Check sheet for the modelled part. Datum: model origin and axes. Units: mm. A direction names the side the tool comes from. Coordinates: 2 decimals unless noted, no trailing zeros. Loops run counter-clockwise (first coordinate to the right, second up) from the corner with the lowest first, then second, coordinate; pieces in that order, holes last. Notation, with made-up numbers: M 26.25,79.25 L 33.25,79.25 A29 ccw 33.25,116.25 Z; hole C -29.75,23 d11. An arc over 180 degrees is marked long. Answer in a Markdown table with one row per item. Add a question column.
Autodesk Inventor part; units mm, degrees
ref_plane "YZ Plane" through (0, 0, 0) normal (1, 0, 0) x (0, 1, 0)
ref_plane "XZ Plane" through (0, 0, 0) normal (0, 1, 0) x (-1, 0, 0)
ref_plane "XY Plane" through (0, 0, 0) normal (0, 0, 1) x (1, 0, 0)
sketch "Boceto1" plane through (0, 0, 0) normal (0, 0, 1) x (1, 0, 0)
  line L0 (-46, -14.91) -> (-46, -35.91)
  line L1 (-44.1, -31.91) -> (-2.9, -31.91)
  line L2 (-1, -35.91) -> (-1, -20.31)
  line L3 (-8.1, 6.6131) -> (-8.1, -14.91)
  line L4 (-44.6, -16.31) -> (-6.4, -16.31)
  line L5 (-2.4, -20.31) -> (-2.4, -30.01)
  line L6 (-2.9, -30.51) -> (-44.1, -30.51)
  line L7 (-44.6, -30.01) -> (-44.6, -16.31)
  arc A0 (-2.4, -20.31) -> (-6.4, -16.31) centre (-6.4, -20.31) ccw
  line L8 (-2.4, -32.41) -> (-2.4, -34.1632)
  line L9 (-3.5, -35.91) -> (-1, -35.91)
  line L10 (-9.5, -14.91) -> (-9.5, 7.7994)
  line L11 (-44.6, -32.41) -> (-44.6, -34.2323)
  line L12 (-43.5, -35.91) -> (-46, -35.91)
  line L13 (-43.5, -35.91) -> (-43.5, -35.4546)
  line L14 (-3.5, -35.91) -> (-3.5, -35.21)
  line L15 (-43.7447, -35.0247) -> (-44.3553, -34.6622)
  line L16 (-3.5, -35.21) -> (-2.6082, -34.5692)
  arc A1 (-2.9, -30.51) -> (-2.4, -30.01) centre (-2.9, -30.01) ccw
  arc A2 (-2.4, -32.41) -> (-2.9, -31.91) centre (-2.9, -32.41) ccw
  arc A3 (-2.6082, -34.5692) -> (-2.4, -34.1632) centre (-2.9, -34.1632) ccw
  arc A4 (-44.6, -30.01) -> (-44.1, -30.51) centre (-44.1, -30.01) ccw
  arc A5 (-44.1, -31.91) -> (-44.6, -32.41) centre (-44.1, -32.41) ccw
  arc A6 (-44.6, -34.2323) -> (-44.3553, -34.6622) centre (-44.1, -34.2323) ccw
  arc A7 (-43.5, -35.4546) -> (-43.7447, -35.0247) centre (-44, -35.4546) ccw
  line L17 (-9.5, 7.7994) -> (-4.75, 8.59)
  line L18 (-4.75, 8.59) -> (0, 7.7994)
  line L19 (-8.1, 6.6131) -> (-4.75, 7.1707)
  line L20 (-4.75, 7.1707) -> (-1.4, 6.6131)
  line L21 (0, 7.7994) -> (0, 0)
  line L22 (0, 0) -> (-1.4, 0)
  line L23 (-1.4, 0) -> (-1.4, 6.6131)
  line L24 (-8.1, -14.91) -> (-6.4, -14.91)
  arc A8 (-1, -20.31) -> (-6.4, -14.91) centre (-6.4, -20.31) ccw
  line L25 (-4.75, 16.5254) -> (-4.75, 0) construction
  line L26 (-38.9, 6.6131) -> (-38.9, -14.91)
  line L27 (-37.5, -14.91) -> (-37.5, 7.7994)
  line L28 (-37.5, 7.7994) -> (-42.25, 8.59)
  line L29 (-42.25, 8.59) -> (-47, 7.7994)
  line L30 (-38.9, 6.6131) -> (-42.25, 7.1707)
  line L31 (-42.25, 7.1707) -> (-45.6, 6.6131)
  line L32 (-47, 7.7994) -> (-47, 0)
  line L33 (-47, 0) -> (-45.6, 0)
  line L34 (-45.6, 0) -> (-45.6, 6.6131)
  line L35 (-42.25, 16.5254) -> (-42.25, 0) construction
  line L36 (-9.5, -14.91) -> (-37.5, -14.91)
  line L37 (-38.9, -14.91) -> (-46, -14.91)
  line L38 (-23.5, 14.1873) -> (-23.5, -36.7854) construction
  point P0 (-44.6, -34.5169)
  point P1 (-43.5, -35.17)
  dimension "d17" = 4
  dimension "d24" = 1.4
  dimension "d50" = 0.7
  dimension "d61" = 0.74
  dimension "d62" = 30.7
  dimension "d63" = 35.7
  dimension "d206" = 1.4
  dimension "d207" = 1.4
  dimension "d210" = 1.4
  dimension "d211" = 1.4
  dimension "d213" = 14.2
  dimension "d214" = 1.4
  dimension "d215" = 1.4
  dimension "d216" = 1.4
  dimension "d217" = 1.4
  dimension "d218" = 45
  dimension "d223" = 5.4
  dimension "d224" = 1.4
  dimension "d225" = 9.5
  dimension "d226" = 4.75
  dimension "d227" = 3.35
  dimension "d228" = 6.7
  dimension "d229" = 44.5
  dimension "d230" = 3.35
  dimension "d231" = 2.5
  dimension "d232" = 2.5
  dimension "d240" = 8.59
  dimension "d241" = 3.35
  dimension "d242" = 99.45
  dimension "d243" = 161.1
  dimension "d246" = 1.4
  dimension "d247" = 1.4
  dimension "d248" = 1.4
  dimension "d253" = 1.4
  dimension "d254" = 1.4
  dimension "d255" = 1.4
  dimension "d256" = 1.4
  dimension "d257" = 8.59
  dimension "d258" = 161.1
  dimension "d259" = 99.45
  dimension "d260" = 22.5
  dimension "d266" = 23.5
  dimension "d267" = 47
  dimension "d268" = 3.35
  dimension "d269" = 9.5
  dimension "d270" = 4.75
  dimension "d271" = 3.35
  dimension "d272" = 6.7
  dimension "d273" = 28
  dimension "d274" = 37.5
  dimension "d275" = 8.5
  dimension "d276" = 8.5
  dimension "d277" = 44.5
  dimension "d278" = 0.5
  dimension "d279" = 14.91
  dimension "d280" = 14.91
  dimension "d283" = 16.5254
  dimension "d284" = 0
  dimension "d285" = 14.1873
  dimension "d286" = 36.7854
  dimension "d287" = 16.5254
  dimension "d288" = 0
extrude "Extrusión1" add sketch "Boceto1" against normal blind 1200
ref_plane "Plano de trabajo2" through (0, 0, -600) normal (0, 0, -1) x (-1, 0, 0)
sketch "Boceto2" plane through (0, 0, 0) normal (1, 0, 0) x (0, 1, 0)
  line L0 (-35.91, 0) -> (-20.31, 0)
  line L1 (-35.91, 0) -> (-35.91, -1200)
  line L2 (-20.31, -1200) -> (-35.91, -1200)
  line L3 (-20.31, 0) -> (-20.31, -1200)
  line L4 (-20.31, 0) -> (-14.91, 0)
  line L5 (-20.31, 0) -> (-20.31, -1200)
  line L6 (-14.91, -1200) -> (-20.31, -1200)
  line L7 (-14.91, 0) -> (-14.91, -1200)
  line L8 (-14.91, 0) -> (6.6131, 0)
  line L9 (-14.91, 0) -> (-14.91, -1200)
  line L10 (6.6131, -1200) -> (-14.91, -1200)
  line L11 (6.6131, 0) -> (6.6131, -1200)
  line L12 (0, 0) -> (7.7994, 0)
  line L13 (0, 0) -> (0, -1200)
  line L14 (7.7994, -1200) -> (0, -1200)
  line L15 (7.7994, 0) -> (7.7994, -1200)
  line L16 (7.7994, 0) -> (8.59, 0)
  line L17 (7.7994, 0) -> (7.7994, -1200)
  line L18 (8.59, -1200) -> (7.7994, -1200)
  line L19 (8.59, 0) -> (8.59, -1200)
  line L20 (-35.91, 0) -> (8.59, -44.5)
  line L21 (8.59, 0) -> (8.59, -44.5)
  line L22 (8.59, 0) -> (-35.91, 0)
  dimension "d291" = 45
extrude "Extrusión2" cut sketch "Boceto2" against normal through all contours L0 L3 L20 | L4 L7 L20 L3 | L8 L13 L20 L7 | L8 L11 L20 L13 | L12 L15 L20 L11 | L16 L19 L20 L15
mirror "Simetría2" about plane through (0, 0, -600) normal (0, 0, -1) of "Extrusión2"
ref_plane "Plano de trabajo4" through (0, 7.7994, 0) normal (0, 1, 0) x (0, 0, -1)
properties part number "SP40-09 MARCO CORREDERA 1200 MM" material "Aluminio"
Q1. Cross-section at A-A (x = -24). Record the cut outline in (y, z), plus the area to 3 significant figures.
Q2. Mould release check, pull along Y, two halves, no side actions. Record for faces 5 (the face through (-38.9, -4, -592)), 6 (the face through (-9.5, -4, -592)), 7 (the face through (-21.65, -15.41, -20.5)): released by +Y, released by -Y, zero draft, split by the parting line, or undercut.
Q3. Thickness scan on L1, parallel to Y at x = -20, z = -735; L2, parallel to X at y = -3.5, z = -724; L3, parallel to X at y = -20.5, z = -1076.5. Record the ranges inside material, lowest first.
Q4. Go/stop test with flat-tipped pins: pin 1 (0.5 mm diameter, centred on y = -33, z = -651, fed in from +X); pin 2 (10 mm diameter, centred on x = -5.5, y = -24, fed in from -Z); pin 3 (3 mm diameter, centred on x = -39, z = -672.5, fed in from -Y). Record where each tip stops, or that it passes through.
Q5. Access from +Z, -Z, +X, -X, +Y, -Y to the whole of each face (thin tool, end or side, straight path). Record for faces 1 (the face through (-21.65, -15.2, -1179.29)), 2 (the face through (-46, -25, -592)), 3 (the face through (-37.5, -4, -592)), 4 (the face through (-23, -30.51, -592)).
Answer key:
| question | item | result |
|---|---|---|
| 1 | outline | M -31.91,-1196 L -30.51,-1194.6 L -30.51,-5.4 L -31.91,-4 Z; M -16.31,-1180.4 L -14.91,-1179 L -14.91,-21 L -16.31,-19.6 Z |
| 1 | area | 3,290 mm^2 |
| 2 | face 5 | undercut |
| 2 | face 6 | zero draft |
| 2 | face 7 | released by +Y |
| 3 | L1 | -31.91 to -30.51, -16.31 to -14.91 |
| 3 | L2 | -38.9 to -37.5, -9.5 to -8.1 |
| 3 | L3 | -46 to -44.6, -2.4 to -1 |
| 4 | pin 1 | x = -1 |
| 4 | pin 2 | z = -1192.01 |
| 4 | pin 3 | y = -31.91 |
| 5 | face 1 | -Z, +X, -X, +Y |
| 5 | face 2 | +Z, -Z, -X, -Y |
| 5 | face 3 | +Z, -Z, +Y |
| 5 | face 4 | +Z, -Z |
